```python
from build123d import *

# Parameters (mm, degrees)
AUFSATZ_LINEAR_AUSTRAGEN1_DEPTH = 12
AUFSATZ_LINEAR_AUSTRAGEN2_DEPTH = 4
SKIZZE3_R                       = 1.85
AUFSATZ_LINEAR_AUSTRAGEN3_DEPTH = 2.7
SKIZZE4_R                       = 0.75
SCHNITT_LINEAR_AUSTRAGEN1_DEPTH = 36.708017307


with BuildPart() as part:
    # Skizze1 → Aufsatz-Linear austragen1 (new body)
    with BuildSketch(Plane(origin=(0, 0, 0), x_dir=(0, 0, -1), z_dir=(1, 0, 0))):
        Polygon((0, 0), (23, 0), (23, 17.5), (27.75, 17.5), (27.75, 19), (23, 19), (23, 21.5), (0, 21.5), (0, 19), (-4.75, 19), (-4.75, 17.5), (0, 17.5), align=None)
    extrude(amount=AUFSATZ_LINEAR_AUSTRAGEN1_DEPTH)

    # Skizze2 → Aufsatz-Linear austragen2 (add)
    with BuildSketch(Plane(origin=(0, 21.5, 0), x_dir=(1, 0, 0), z_dir=(0, 1, 0))):
        with BuildLine():
            Line((3.744418815, 15.078125), (0.631716779, 8.5659375))
            ThreePointArc((0.631716779, 8.5659375), (6, 0.05), (11.368283221, 8.5659375))
            Line((11.368283221, 8.5659375), (8.255581185, 15.078125))
            ThreePointArc((8.255581185, 15.078125), (6, 16.5), (3.744418815, 15.078125))
        make_face()
    extrude(amount=AUFSATZ_LINEAR_AUSTRAGEN2_DEPTH)

    # Skizze3 → Aufsatz-Linear austragen3 (add)
    with BuildSketch(Plane(origin=(0, 25.5, 0), x_dir=(1, 0, 0), z_dir=(0, 1, 0))):
        with Locations(Location((6, 6, 0), (0, 0, 90))):
            Circle(SKIZZE3_R)
    extrude(amount=AUFSATZ_LINEAR_AUSTRAGEN3_DEPTH)

    # Skizze4 → Schnitt-Linear austragen1 (cut, through all)
    with BuildSketch(Plane(origin=(0, 19, 0), x_dir=(1, 0, 0), z_dir=(0, 1, 0))):
        with Locations(Location((6, -2.5, 0), (0, 0, 270))):
            Circle(SKIZZE4_R)
        with Locations(Location((6, 25.5, 0), (0, 0, 270))):
            Circle(SKIZZE4_R)
    extrude(amount=-SCHNITT_LINEAR_AUSTRAGEN1_DEPTH, mode=Mode.SUBTRACT)


solid = part.part
```
Geometry check sheet. Reference: the model listing, model coordinates, mm. A direction names the side the tool comes from. Give positions to 0.01 mm unless a question says otherwise; leave off trailing zeros. Order: outer loops, then holes, each group sorted by start corner. A loop starts at its lowest first (then second) coordinate and runs counter-clockwise, first axis right, second up.
1. Section check B-B, the plane z = -25.5. Enter the section's corners in (x, y), and give its area (4 significant figures).
2. Section check C-C, the plane z = -6. Enter the section's corners in (x, y).
3. Section check A-A, the plane x = 6. Enter the section's corners in (y, z), and give its area (3 significant figures).
4. Release check for a two-part mould opening along X. For faces 1 (the face through (6.03, 18.26, -26.25)), 2 (the face through (6, 9, 0)), 3 (the face through (5.832, 23.472, -0.052)), 4 (the face through (5.71, 18.26, 3.19)) record: pulls with the +X half, pulls with the -X half, needs draft (parallel to the pull), parting line crosses it, or undercut.
5. Gauge pin test, flat ends, axial feed: pin 1 Ø2.5 at (x, z) = (6, 2.5) entering from +Y; pin 2 Ø1 at (x, z) = (6.5, -15) entering from +Y; pin 3 Ø1.4 at (x, z) = (6.5, 3) entering from -Y; pin 4 Ø1.2 at (x, z) = (6, -25.5) entering from -Y. Record the tip position at first contact, or that the pin passes through.
6. Section check D-D, the plane x = 1.25. Enter the section's corners in (y, z), and give its area (3 significant figures).
7. Access from +Z, -Z, +X, -X, +Y, -Y to the whole of each face (thin tool, end or side, straight path). Record for faces 5 (the face through (5.9, 17.5, -26.4)), 6 (the face through (6, 23.5, -16.5)), 7 (the face through (6, 20, -23)), 8 (the face through (9.83, 23.47, -11.78)), 9 (the face through (6, 19, 1)).
8. Thickness scan on L1, parallel to X at y = 18.55, z = -25.5; L2, parallel to Z at x = 1, y = 16.25; L3, parallel to Y at x = 6.5, z = -22. Record the ranges inside material, lowest first.
Values follow:
1. outline: (0, 17.5) - (5.25, 17.5) - (5.25, 19) - (0, 19) - close; (6.75, 17.5) - (12, 17.5) - (12, 19) - (6.75, 19) - close
1. area: 15.75 mm2
2. outline: (0, 0) - (12, 0) - (12, 21.5) - (11.95, 21.5) - (11.95, 25.5) - (7.85, 25.5) - (7.85, 28.2) - (4.15, 28.2) - (4.15, 25.5) - (0.05, 25.5) - (0.05, 21.5) - (0, 21.5) - close
3. outline: (0, -23) - (17.5, -23) - (17.5, -24.75) - (19, -24.75) - (19, -23) - (21.5, -23) - (21.5, -16.5) - (25.5, -16.5) - (25.5, -7.85) - (28.2, -7.85) - (28.2, -4.15) - (25.5, -4.15) - (25.5, -0.05) - (21.5, -0.05) - (21.5, 0) - (19, 0) - (19, 1.75) - (17.5, 1.75) - (17.5, 0) - (0, 0) - close; (17.5, -27.75) - (19, -27.75) - (19, -26.25) - (17.5, -26.25) - close; (17.5, 3.25) - (19, 3.25) - (19, 4.75) - (17.5, 4.75) - close
3. area: 580 mm2
4. face 1: undercut
4. face 2: needs draft
4. face 3: parting line crosses it
4. face 4: undercut
5. pin 1: stops at y = 19
5. pin 2: stops at y = 25.5
5. pin 3: stops at y = 17.5
5. pin 4: passes through
6. outline: (0, -23) - (17.5, -23) - (17.5, -27.75) - (19, -27.75) - (19, -23) - (21.5, -23) - (21.5, -9.86) - (25.5, -9.86) - (25.5, -2.42) - (21.5, -2.42) - (21.5, 0) - (19, 0) - (19, 4.75) - (17.5, 4.75) - (17.5, 0) - (0, 0) - close
6. area: 539 mm2
7. face 5: -Z, +X, -X, -Y
7. face 6: -Z, +Y
7. face 7: -Z, +X, -X, +Y
7. face 8: -Z, +X, +Y
7. face 9: +Z, +X, -X, +Y
8. L1: x = 0 to 5.25, 6.75 to 12
8. L2: z = -23 to 0
8. L3: y = 0 to 21.5
